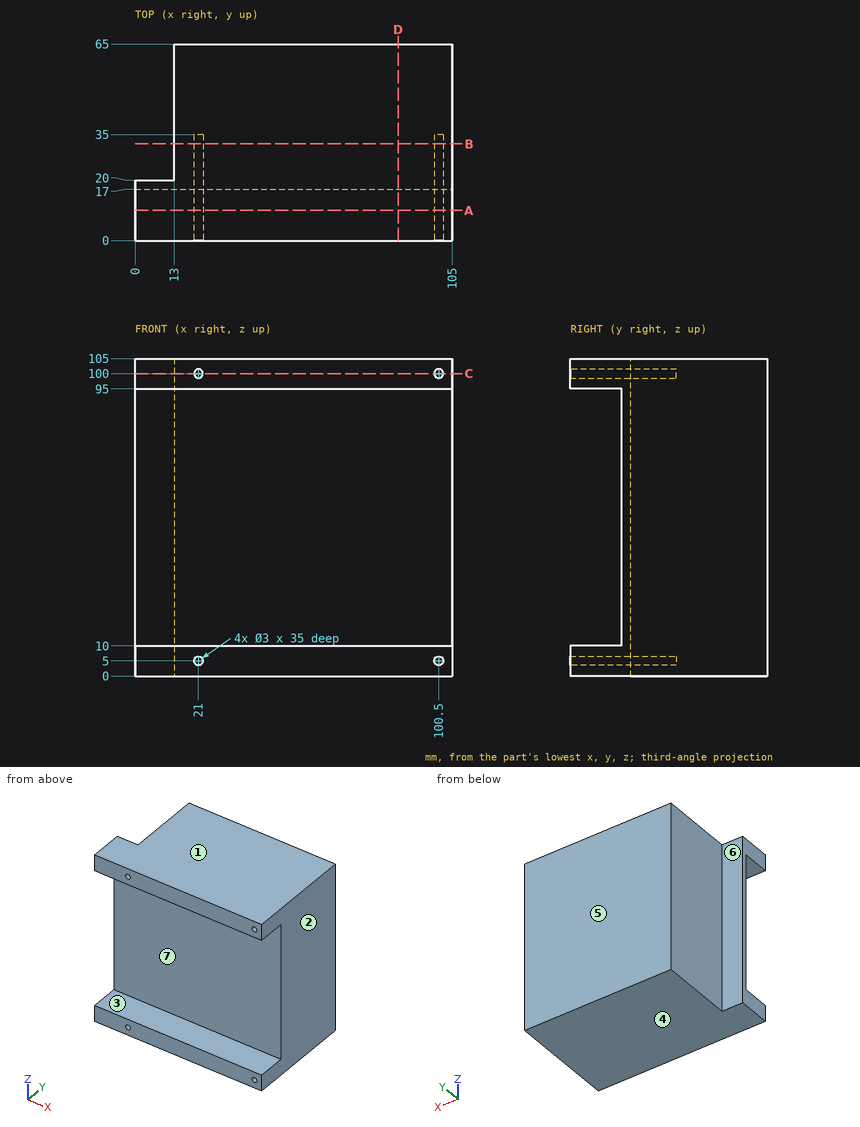
Study the drawing (mm; zero at the part's minimum x, y, z) and answer. A direction names the side the tool comes from. Coordinates: 2 decimals unless noted, no trailing zeros. Loops run counter-clockwise (first coordinate to the right, second up) from the corner with the lowest first, then second, coordinate; pieces in that order, holes last. Notation, with made-up numbers: (-18, 31) -> (25, 31) arc R19 cw to (25, 68) -> close; hole circle Ø3 at (23.5, 64.25). An arc over 180 degrees is marked (long way). Write item = value, one per line. Start each with the question number.
1) The mould has two halves that part along Z. Classify the marked faces 1, 2, 3 and 4: pulls with the +Z half, pulls with the -Z half, needs draft (parallel to the pull), parting line crosses it, or undercut.
2) The part is cut by section A-A, the plane y = 10. Determine the outline of the cut face in (x, z), plus the area to 3 significant figures.
3) The part is cut by section D-D, the plane x = 87. Determine the outline of the cut face in (y, z).
4) For the marked faces 5, 6 and 7, determine the directions among +Z, -Z, +X, -X, +Y, -Y from which every point of the face is accessible in a straight line to the end or side of a thin tool.
5) Given P1, Ø22.5, axis at y = 37.5, z = 45, coming from the -X side; P2, Ø2.5, axis at x = 21.5, z = 100.5, coming from the -Y side; P3, Ø1.5, axis at x = 28, z = 62, coming from the -Y side; P4, Ø1.8, axis at x = 21, z = 5, coming from the -Y side, each flat-ended and moving along its own axis, determine where each tip first touches the part or whether it passes through.
6) Find the intervals of material crossed by L1, parallel to Z at x = 100.5, y = 8; L2, parallel to X at y = 25, z = 5; L3, parallel to Z at x = 38, y = 10, in increasing order. Write a range as from..to.
7) The part is cut by section B-B, the plane y = 32. Determine the outline of the cut face in (x, z).
8) The part is cut by section C-C, the plane z = 100. Determine the outline of the cut face in (x, y), plus the area to 3 significant figures.
Result:
q1.face_1 = pulls with the +Z half
q1.face_2 = needs draft
q1.face_3 = undercut
q1.face_4 = pulls with the -Z half
q2.outline = (0, 0) -> (105, 0) -> (105, 10) -> (0, 10) -> close; (0, 95) -> (105, 95) -> (105, 105) -> (0, 105) -> close; hole circle Ø3 at (21, 5); hole circle Ø3 at (21, 100); hole circle Ø3 at (100.5, 5); hole circle Ø3 at (100.5, 100)
q2.area = 2,070 mm²
q3.outline = (0, 0) -> (65, 0) -> (65, 105) -> (0, 105) -> (0, 95) -> (17, 95) -> (17, 10) -> (0, 10) -> close
q4.face_5 = +Z, -Z, +X, -X, +Y
q4.face_6 = +Z, -Z, -X, +Y
q4.face_7 = +X, -X, -Y
q5.P1 = 13
q5.P2 = 0
q5.P3 = 17
q5.P4 = 35
q6.L1 = 0..3.5, 6.5..10, 95..98.5, 101.5..105
q6.L2 = 13..19.5, 22.5..99, 102..105
q6.L3 = 0..10, 95..105
q7.outline = (13, 0) -> (105, 0) -> (105, 105) -> (13, 105) -> close; hole circle Ø3 at (21, 5); hole circle Ø3 at (21, 100); hole circle Ø3 at (100.5, 5); hole circle Ø3 at (100.5, 100)
q8.outline = (0, 0) -> (19.5, 0) -> (19.5, 35) -> (22.5, 35) -> (22.5, 0) -> (99, 0) -> (99, 35) -> (102, 35) -> (102, 0) -> (105, 0) -> (105, 65) -> (13, 65) -> (13, 20) -> (0, 20) -> close
q8.area = 6,030 mm²
